from build123d import *

# Parameters (mm, degrees)
SKETCH2_W             = 23.81
SKETCH2_H             = 10.7125
SKETCH2_W_2           = 19.0525
SKETCH2_W_3           = 11.11
SKETCH2_W_4           = 9.39
SKETCH2_W_5           = 6.35
SKETCH2_W_6           = 1.725
SKETCH2_W_7           = 1.585
SKETCH2_W_8           = 6.3525
BOSS_EXTRUDE1_DEPTH   = 12.7
M4X0_7_TAPPED_HOLE1_D = 3.3
FILLET1_R             = 5


with BuildPart() as part:
    # Sketch2 → Boss-Extrude1 (new body)
    with BuildSketch(Plane(origin=(0, 0, 0), x_dir=(1, 0, 0), z_dir=(0, 1, 0))):
        with Locations((24.605, 66.53125)):
            Rectangle(SKETCH2_W, SKETCH2_H)
        with Locations((3.17375, 66.53125)):
            Rectangle(SKETCH2_W_2, SKETCH2_H)
        with BuildLine():
            Line((0, 22.6), (1.585, 22.6))
            Line((1.585, 22.6), (3.31, 22.6))
            Line((3.31, 22.6), (12.7, 22.6))
            Line((12.7, 22.6), (12.7, 27.6))
            ThreePointArc((12.7, 27.6), (-1.5875, 41.8875), (12.7, 56.175))
            Line((12.7, 56.175), (12.7, 61.175))
            Line((12.7, 61.175), (-6.3525, 61.175))
            Line((-6.3525, 61.175), (-6.3525, 22.6))
            Line((-6.3525, 22.6), (0, 22.6))
        make_face()
        with BuildLine():
            Line((12.7, 22.6), (23.81, 22.6))
            Line((23.81, 22.6), (30.16, 22.6))
            Line((30.16, 22.6), (36.51, 22.6))
            Line((36.51, 22.6), (36.51, 61.175))
            Line((36.51, 61.175), (12.7, 61.175))
            Line((12.7, 61.175), (12.7, 56.175))
            ThreePointArc((12.7, 56.175), (22.802788136, 51.990288136), (26.9875, 41.8875))
            ThreePointArc((26.9875, 41.8875), (22.802788136, 31.784711864), (12.7, 27.6))
            Line((12.7, 27.6), (12.7, 22.6))
        make_face()
        with Locations((18.255, 17.24375)):
            Rectangle(SKETCH2_W_3, SKETCH2_H)
        with Locations((8.005, 17.24375)):
            Rectangle(SKETCH2_W_4, SKETCH2_H)
        with Locations((26.985, 17.24375)):
            Rectangle(SKETCH2_W_5, SKETCH2_H)
        with Locations((33.335, 17.24375)):
            Rectangle(SKETCH2_W_5, SKETCH2_H)
        with Locations((2.4475, 17.24375)):
            Rectangle(SKETCH2_W_6, SKETCH2_H)
        with Locations((0.7925, 17.24375)):
            Rectangle(SKETCH2_W_7, SKETCH2_H)
        with Locations((-3.17625, 17.24375)):
            Rectangle(SKETCH2_W_8, SKETCH2_H)
        Polygon((36.51, 22.6), (36.51, 11.8875), (41.2725, 11.8875), (41.2725, 71.8875), (36.51, 71.8875), (36.51, 61.175), align=None)
    extrude(amount=BOSS_EXTRUDE1_DEPTH)

    # M4x0.7 Tapped Hole1 (through all)
    with Locations(Plane(origin=(41.2725, 0, 0), x_dir=(0, 0, -1), z_dir=(1, 0, 0))):
        with Locations((63.8875, 6.35), (19.8875, 6.35)):
            Hole(M4X0_7_TAPPED_HOLE1_D / 2)

    # Fillet1
    fillet1_edges = [part.edges().sort_by_distance(p)[0] for p in [
        (17.46, 0, -11.8875),
        (17.46, 12.7, -11.8875),
        (17.46, 12.7, -71.8875),
        (17.46, 0, -71.8875),
    ]]
    fillet(fillet1_edges, radius=FILLET1_R)


solid = part.part
Work out the finished part from the listing and answer in its coordinate system (mm). Coordinates: 2 decimals unless noted, no trailing zeros. Order: outer loops, then holes, each group sorted by start corner. A loop starts at its lowest first (then second) coordinate and runs counter-clockwise, first axis right, second up. Notation, with made-up numbers: (-35.75, 64.5) - (14.25, 64.5) arc R31 ccw to (14.25, 90.5) - close; hole circle Ø4 at (71.5, 72.5). An arc over 180 degrees is marked (long way). Put each result on its own line as item: value. Start each with the question number.
1) Find section D-D (x = 30). Give the vertices of the cut face in (y, z), plus the area to 3 significant figures.
2) For a pull along Z with two mould halves and no side action, classify faces 1 (the cylindrical face through (17.793, 11.274, -13.391)), 2 (the cylindrical face through (17.127, 5.718, -62.363)), 3 (the flat face through (28, 12.7, -42)) as released by +Z, released by -Z, zero draft, split by the parting line, or undercut.
3) Find section C-C (z = -30.5). Give the vertices of the cut face in (x, y), plus the area to 3 significant figures.
4) Find section B-B (x = 16.5). Give the vertices of the cut face in (y, z), plus the area to 3 significant figures.
5) Find the intervals of material crossed by line 1 (Z direction, x = 32, y = 6.5); line 2 (Z direction, x = 2, y = 7); line 3 (X direction, y = 10.25, z = -45), in increasing order. Write a range as from..to.
6) Find section A-A (y = 6.35). Give the vertices of the cut face in (x, z) (1 decimal), plus the area to 3 significant figures.
7) A flat-ended cylindrical pin translates along its axis: pin 1 (3 mm diameter, centred on x = 35, y = 3.5, fed in from -Z). Find the tip coordinate at first contact, or state that the pin passes through.
Results list:
1. outline: (0, -66.89) arc R5 ccw to (5, -71.89) - (7.7, -71.89) arc R5 ccw to (12.7, -66.89) - (12.7, -16.89) arc R5 ccw to (7.7, -11.89) - (5, -11.89) arc R5 ccw to (0, -16.89) - close; hole circle Ø3.3 at (6.35, -63.89); hole circle Ø3.3 at (6.35, -19.89)
1. area: 723 mm^2
2. face 1: released by +Z
2. face 2: undercut
2. face 3: zero draft
3. outline: (-6.35, 0) - (4.07, 0) - (4.07, 12.7) - (-6.35, 12.7) - close; (21.33, 0) - (41.27, 0) - (41.27, 12.7) - (21.33, 12.7) - close
3. area: 386 mm^2
4. outline: (0, -66.89) arc R5 ccw to (5, -71.89) - (7.7, -71.89) arc R5 ccw to (12.7, -66.89) - (12.7, -55.66) - (0, -55.66) - close; (0, -28.11) - (12.7, -28.11) - (12.7, -16.89) arc R5 ccw to (7.7, -11.89) - (5, -11.89) arc R5 ccw to (0, -16.89) - close; hole circle Ø3.3 at (6.35, -63.89); hole circle Ø3.3 at (6.35, -19.89)
4. area: 374 mm^2
5. line 1: z = -71.89..-65.53, -62.24..-21.53, -18.24..-11.89
5. line 2: z = -71.89..-65.4, -62.37..-51.36, -32.42..-21.4, -18.37..-11.89
5. line 3: x = -6.35..-1.24, 26.64..41.27
6. outline: (-6.4, -71.9) - (41.3, -71.9) - (41.3, -65.5) - (-6.4, -65.5) - close; (-6.4, -62.2) - (41.3, -62.2) - (41.3, -21.5) - (-6.4, -21.5) - close; (-6.4, -18.2) - (41.3, -18.2) - (41.3, -11.9) - (-6.4, -11.9) - close; hole circle Ø28.6 at (12.7, -41.9)
6. area: 1,900 mm^2
7. pin 1: stops at z = -71.89
